Autodesk Inventor part; units mm, degrees
ref_plane "YZ Plane" through (0, 0, 0) normal (1, 0, 0) x (0, 1, 0)
ref_plane "XZ Plane" through (0, 0, 0) normal (0, 1, 0) x (-1, 0, 0)
ref_plane "XY Plane" through (0, 0, 0) normal (0, 0, 1) x (1, 0, 0)
sketch "Sketch1" plane through (0, 0, 0) normal (1, 0, 0) x (0, 1, 0)
  line L0 (0, 0) -> (3.875, 0)
  line L1 (3.875, 0) -> (3.875, 3.2)
  line L2 (3.875, 3.2) -> (4.25, 3.2)
  line L3 (4.25, 3.2) -> (4.8, 80.3)
  line L4 (4.8, 80.3) -> (4.325, 80.3)
  line L5 (0, 0) -> (0, 129.1)
  line L6 (4.325, 80.3) -> (4.325, 82.8)
  line L7 (4.325, 82.8) -> (4.4, 82.8)
  line L8 (4.4, 82.8) -> (4.4, 85.8)
  line L9 (4.4, 85.8) -> (4.25, 85.8)
  line L10 (4.25, 85.8) -> (4, 110.3)
  line L11 (4, 110.3) -> (3.375, 110.3)
  line L12 (3.375, 110.3) -> (0.2, 129.1)
  line L13 (0.2, 129.1) -> (0, 129.1)
  dimension "d0" = 3.875
  dimension "d1" = 3.2
  dimension "d2" = 4.25
  dimension "d3" = 4.8
  dimension "d4" = 80.3
  dimension "d5" = 4.325
  dimension "d6" = 2.5
  dimension "d7" = 3
  dimension "d8" = 4.4
  dimension "d9" = 4.25
  dimension "d10" = 4
  dimension "d11" = 3.375
  dimension "d12" = 129.1
  dimension "d13" = 30
  dimension "d15" = 0.2
revolve "Revolution1" add sketch "Sketch1" angle 360 about axis through (0, 0, 0) along (0, 0, 1)
properties part number "pen"
CAD build for the part. Positions are in the model's coordinates, mm. A direction names the side the tool comes from. Give positions to 0.01 mm unless a question says otherwise; leave off trailing zeros. Order: outer loops, then holes, each group sorted by start corner. A loop starts at its lowest first (then second) coordinate and runs counter-clockwise, first axis right, second up.
(1) Saw through at A-A, the plane z = 77. Give the cut face in (x, y), then the cut area to 3 significant figures.
(2) Saw through at B-B, the plane z = 13. Give the cut face in (x, y).
(3) Flat gauge pins, fed straight in: pin 1 (2 mm diameter, centred on x = 1, z = 32, fed in from -Y); pin 2 (2 mm diameter, centred on x = -2.5, z = 18, fed in from +Y); pin 3 (1 mm diameter, centred on x = 1, z = 113.5, fed in from +Y). Where does each tip first touch, or does it go through?
(4) Drill centre lines: L1, parallel to Y at x = -1.5, z = 42; L2, parallel to Z at x = 1, y = 3.5; L3, parallel to Y at x = -2.25, z = 79. Where is each one in solid material? Low to high.
(5) Tool access for faces 1 (the cylindrical face through (-3.842, -0.504, 1.622)), 2 (the conical face through (-4.03, -0.89, 97.88)), 3 (the flat face through (0, 0, 0)): list every direction of +Z, -Z, +X, -X, +Y, -Y with a clear straight run to the whole face (end or side of a thin tool).
Results found:
1. outline: circle Ø9.55 at (0, 0)
1. area: 71.7 mm2
2. outline: circle Ø8.64 at (0, 0)
3. pin 1: stops at y = -4.46
3. pin 2: stops at y = 4.09
3. pin 3: stops at y = 2.82
4. L1: y = -4.27 to 4.27
4. L2: z = 0 to 110.3
4. L3: y = -4.23 to 4.23
5. face 1: -Z
5. face 2: +Z
5. face 3: -Z, +X, -X, +Y, -Y
